```python
from build123d import *

# Parameters (mm, degrees)
F1_DEPTH = 5.8


with BuildPart() as f1:
    # F0 (on Front) → F1 (new body)
    with BuildSketch(Plane.XZ):
        Polygon((87.5, 62.3), (87.5, 67.3), (62.5, 67.3), (62.5, 73.65), (20.2, 73.65), (20.2, 67.3), (-20.2, 67.3), (-20.2, 73.65), (-62.5, 73.65), (-62.5, 67.3), (-87.5, 67.3), (-87.5, 62.3), (-93.85, 62.3), (-93.85, 20.3), (-87.5, 20.3), (-87.5, -20.3), (-93.85, -20.3), (-93.85, -62.3), (-87.5, -62.3), (-87.5, -67.3), (-62.5, -67.3), (-62.5, -73.65), (-20.2, -73.65), (-20.2, -67.3), (20.2, -67.3), (20.2, -73.65), (62.5, -73.65), (62.5, -67.3), (87.5, -67.3), (87.5, -62.3), (93.85, -62.3), (93.85, -20.3), (87.5, -20.3), (87.5, 20.3), (93.85, 20.3), (93.85, 62.3), align=None)
        with BuildLine():
            ThreePointArc((-2.48414, -16.414051), (-3.011348, -17.686843), (-4.28414, -18.214051))
            Line((-4.28414, -18.214051), (-18.722851, -18.214053))
            ThreePointArc((-18.722851, -18.214053), (-19.995643, -17.686845), (-20.522851, -16.414053))
            Line((-20.522851, -16.414053), (-20.522851, 2.993572))
            ThreePointArc((-20.522851, 2.993572), (-19.995643, 4.266364), (-18.722851, 4.793572))
            Line((-18.722851, 4.793572), (-4.28414, 4.79357))
            ThreePointArc((-4.28414, 4.79357), (-3.011348, 4.266362), (-2.48414, 2.99357))
            Line((-2.48414, 2.99357), (-2.48414, -3.186868))
            Line((-2.48414, -3.186868), (-6.911026, -3.186868))
            Line((-6.911026, -3.186868), (-6.911026, 1.14975))
            Line((-6.911026, 1.14975), (-16.095965, 1.14975))
            Line((-16.095965, 1.14975), (-16.095965, -14.57023))
            Line((-16.095965, -14.57023), (-6.911026, -14.57023))
            Line((-6.911026, -14.57023), (-6.911026, -9.962669))
            Line((-6.911026, -9.962669), (-2.48414, -9.962669))
            Line((-2.48414, -9.962669), (-2.48414, -16.414051))
        make_face(mode=Mode.SUBTRACT)
        Polygon((4.802941, -18.214051), (0.285788, -18.153826), (8.05544, 4.793572), (12.753269, 4.793572), (20.522851, -18.153826), (15.975515, -18.214051), (10.374172, -0.235564), align=None, mode=Mode.SUBTRACT)
        Polygon((-17.285935, 7.171967), (-20.494564, 7.171967), (-20.494564, 18.214053), (-17.025802, 18.214053), (-14.539873, 12.288281), (-12.126241, 18.214053), (-8.686399, 18.214053), (-8.686399, 7.171967), (-11.851649, 7.171967), (-11.851649, 12.100447), (-13.253599, 7.648853), (-15.884055, 7.648853), (-17.285935, 12.100447), align=None, mode=Mode.SUBTRACT)
        Polygon((-3.960774, 11.536803), (-3.960774, 7.171967), (-7.227172, 7.171967), (-7.227172, 18.214053), (1.675946, 18.214053), (1.675946, 15.554749), (-3.960774, 15.554749), (-3.960774, 14.051651), (0.404062, 14.051651), (0.404062, 11.536803), align=None, mode=Mode.SUBTRACT)
        Polygon((4.204833, 7.171967), (0.880667, 7.200886), (4.696249, 18.214053), (8.1794, 18.214053), (11.995052, 7.200886), (8.641967, 7.171967), (6.43063, 14.687593), align=None, mode=Mode.SUBTRACT)
    extrude(amount=F1_DEPTH)


solid = f1.part
```
Verification items for the finished model (mm, model axes). A direction names the side the tool comes from. Coordinates: 2 decimals unless noted, no trailing zeros. Answer as a JSON object with one key per item and string values. Group by question number.
(1) Material ranges on line 1 (Z direction, x = -1.5, y = -1.9); line 2 (Z direction, x = -19, y = -0.45); line 3 (X direction, y = -4.15, z = 2.5), recorded low to high.
(2) Tool access check on faces 4 (the face through (-87.5, -3, 65)), 5 (the face through (-2, -3, 14.052)), 6 (the face through (62.5, -3, -71)). Record the directions out of +Z, -Z, +X, -X, +Y, -Y that give a thin tool (end or side, any length) a straight path to the whole face; none if there is none.
(3) Gauge pin test, flat ends, axial feed: pin 1 (2.5 mm diameter, centred on x = 10.5, y = -2, fed in from -Z); pin 2 (3 mm diameter, centred on y = -4, z = 17, fed in from -X); pin 3 (3 mm diameter, centred on y = -3.5, z = -72, fed in from -X); pin 4 (1 mm diameter, centred on x = -34, z = 39.5, fed in from +Y). Record the tip position at first contact, or that the pin passes through.
(4) Release check for a two-part mould opening along X. For faces 1 (the face through (-20.495, -3, 13)), 2 (the face through (93.85, -3, 41)), 3 (the face through (91, -3, 62.3)) record: +X half, -X half, draft (parallel to the pull), parting line (faces both ways), or undercut.
(5) Cross-section at A-A, the plane y = -3.5. State how many separate pieces and enclosed holes the cut face has, and give its area (3 significant figures).
Reply:
{
 "1": {"line 1": "-67.3 to 11.54, 14.05 to 15.55, 18.21 to 67.3", "line 2": "-67.3 to -18.19, 4.77 to 7.17, 18.21 to 67.3", "line 3": "-87.5 to -20.52, -2.48 to 7.28, 13.53 to 87.5"},
 "2": {"face 4": "+Z, -X, +Y, -Y", "face 5": "+Y, -Y", "face 6": "-Z, +X, +Y, -Y"},
 "3": {"pin 1": "z = -67.3", "pin 2": "x = -87.5", "pin 3": "x = -62.5", "pin 4": "y = 0"},
 "4": {"face 1": "undercut", "face 2": "+X half", "face 3": "draft"},
 "5": {"separate pieces": "1", "enclosed holes": "5", "area": "25,000 mm²"}
}
